Here's how the part is built. I have some questions about the finished solid (model axes, mm). A direction names the side the tool comes from. Coordinates: 2 decimals unless noted, no trailing zeros. Loops run counter-clockwise (first coordinate to the right, second up) from the corner with the lowest first, then second, coordinate; pieces in that order, holes last. Notation, with made-up numbers: (80, 5) - (86, 5) arc R8 ccw to (86, 11) - close; hole circle Ø7 at (-18.5, 7.5). An arc over 180 degrees is marked (long way). Use a Markdown table: item, result.
```python
from build123d import *

# Parameters (mm, degrees)
SKETCH1_W           = 57.15
SKETCH1_H           = 127
BOSS_EXTRUDE1_DEPTH = 6.35
SKETCH2_W           = 50.8
SKETCH2_H           = 120.65
CUT_EXTRUDE1_DEPTH  = 1.5875
SKETCH3_W           = 38.1
SKETCH3_H           = 44.45
CUT_EXTRUDE2_DEPTH  = 4.7625


with BuildPart() as part:
    # Sketch1 → Boss-Extrude1 (new, symmetric)
    with BuildSketch(Plane.XY):
        Rectangle(SKETCH1_W, SKETCH1_H)
    extrude(amount=BOSS_EXTRUDE1_DEPTH, both=True)

    # Sketch2 → Cut-Extrude1 (cut, symmetric)
    with BuildSketch(Plane.XY):
        with Locations((0, 3.175)):
            Rectangle(SKETCH2_W, SKETCH2_H)
    extrude(amount=CUT_EXTRUDE1_DEPTH, both=True, mode=Mode.SUBTRACT)

    # Sketch3 → Cut-Extrude2 (cut, symmetric)
    with BuildSketch(Plane.XY):
        with Locations((0, 41.275)):
            Rectangle(SKETCH3_W, SKETCH3_H)
    extrude(amount=CUT_EXTRUDE2_DEPTH, both=True, mode=Mode.SUBTRACT)


solid = part.part
```
Q1. I want a section at B-B, the plane x = 16.5. Write out the boundary of the cut face in (y, z), then the cut area to 3 significant figures.
Check values:
| item | result |
|---|---|
| outline | (-63.5, -6.35) - (63.5, -6.35) - (63.5, -4.76) - (19.05, -4.76) - (19.05, -1.59) - (-57.15, -1.59) - (-57.15, 1.59) - (19.05, 1.59) - (19.05, 4.76) - (63.5, 4.76) - (63.5, 6.35) - (-63.5, 6.35) - close |
| area | 948 mm^2 |
Q2. Please list where these lines run through material, in increasing order: L1, parallel to Z at x = -25, y = -27.5; L2, parallel to X at y = 4.5, z = -1.25 (3 decimals); L3, parallel to Z at x = 3, y = 37. Write a range as from..to.
Check values:
| item | result |
|---|---|
| L1 | -6.35..-1.59, 1.59..6.35 |
| L2 | -28.575..-25.4, 25.4..28.575 |
| L3 | -6.35..-4.76, 4.76..6.35 |
Q3. I want a section at C-C, the plane z = 0. Write out the boundary of the cut face in (x, y) (3 decimals).
Check values:
| item | result |
|---|---|
| outline | (-28.575, -63.5) - (28.575, -63.5) - (28.575, 63.5) - (25.4, 63.5) - (25.4, -57.15) - (-25.4, -57.15) - (-25.4, 63.5) - (-28.575, 63.5) - close |
Q4. Will these pins go through, and if not, where does the flat tip stop? P1, Ø2.5, axis at x = -2, z = -3, coming from the +Y side; P2, Ø1.6, axis at x = 8, z = -0.5, coming from the +Y side.
Check values:
| item | result |
|---|---|
| P1 | y = 19.05 |
| P2 | y = -57.15 |
Q5. Which directions (+Z, -Z, +X, -X, +Y, -Y) give clear straight access to the entire face, cutting with the end or side of a thin tool? Please do faces 4 (the face through (-28.575, -1, 0)), 5 (the face through (19.05, 41, 3)).
Check values:
| item | result |
|---|---|
| face 4 | +Z, -Z, -X, +Y, -Y |
| face 5 | +Y |
Q6. If we mould it in two halves opening along Z, with no side actions, what happens to faces 1 (the face through (0, -63.5, 0)), 2 (the face through (0, 1, 6.35)), 3 (the face through (-25.4, 2, 0))? For each: pulls with the +Z half, pulls with the -Z half, needs draft (parallel to the pull), parting line crosses it, or undercut.
Check values:
| item | result |
|---|---|
| face 1 | needs draft |
| face 2 | pulls with the +Z half |
| face 3 | undercut |
